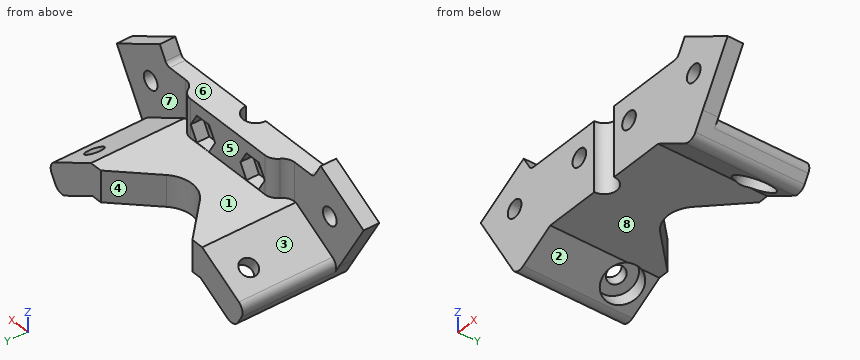
from build123d import *

# Parameters (mm, degrees)
SKETCH1_R                = 2.75
BOSS_EXTRUDE1_DEPTH      = 5
BOSS_EXTRUDE2_DEPTH      = 30
BOSS_EXTRUDE2_DEPTH_BACK = 5
BOSS_EXTRUDE3_DEPTH      = 12.320508
SKETCH5_R                = 4
CUT_EXTRUDE1_DEPTH       = 28.320508076
SKETCH7_R                = 2.75
CUT_EXTRUDE3_DEPTH       = 51.510942144
CUT_EXTRUDE4_START       = -4
SKETCH8_R                = 6
CUT_EXTRUDE4_DEPTH       = 47.510942144
SKETCH9_R                = 2.75
CUT_EXTRUDE5_DEPTH       = 10
CUT_EXTRUDE6_DEPTH       = 4
FILLET2_R                = 3


with BuildPart() as part:
    # Sketch1 → Boss-Extrude1 (new body)
    with BuildSketch(Plane(origin=(0, 0, 0), x_dir=(1, 0, 0), z_dir=(0, 1, 0))):
        with BuildLine():
            Line((-39.711904038, 0), (39.711904038, 0))
            Line((39.711904038, 0), (49.711904038, -17.320508076))
            Line((49.711904038, -17.320508076), (32.391395962, -27.320508076))
            Line((32.391395962, -27.320508076), (30.081994885, -23.320508076))
            ThreePointArc((30.081994885, -23.320508076), (29.349944078, -22.588457268), (28.349944078, -22.320508076))
            Line((28.349944078, -22.320508076), (-28.349944078, -22.320508076))
            ThreePointArc((-28.349944078, -22.320508076), (-29.349944078, -22.588457268), (-30.081994885, -23.320508076))
            Line((-30.081994885, -23.320508076), (-32.391395962, -27.320508076))
            Line((-32.391395962, -27.320508076), (-49.711904038, -17.320508076))
            Line((-49.711904038, -17.320508076), (-39.711904038, 0))
        make_face()
        with Locations(Location((-36.05165, -13.660254038, 0), (0, 0, 270))):  # turned: the seam where the file's is
            Circle(SKETCH1_R, mode=Mode.SUBTRACT)
        with Locations(Location((36.05165, -13.660254038, 0), (0, 0, 270))):  # turned: the seam where the file's is
            Circle(SKETCH1_R, mode=Mode.SUBTRACT)
    extrude(amount=BOSS_EXTRUDE1_DEPTH)

    # Sketch2 → Boss-Extrude2 (add, two sides)
    with BuildSketch(Plane(origin=(0, 5, 0), x_dir=(1, 0, 0), z_dir=(0, 1, 0))) as boss_extrude2_sk:
        with BuildLine():
            Line((-39.711904038, 0), (-22.391395962, -10))
            Line((-22.391395962, -10), (22.391395962, -10))
            Line((22.391395962, -10), (39.711904038, 0))
            Line((39.711904038, 0), (36.711904038, 5.196152423))
            ThreePointArc((36.711904038, 5.196152423), (34.890284962, 6.593929902), (32.613827826, 6.294228634))
            Line((32.613827826, 6.294228634), (21.711904038, 0))
            Line((21.711904038, 0), (-21.711904038, 0))
            Line((-21.711904038, 0), (-32.613827826, 6.294228634))
            ThreePointArc((-32.613827826, 6.294228634), (-34.890284962, 6.593929902), (-36.711904038, 5.196152423))
            Line((-36.711904038, 5.196152423), (-39.711904038, 0))
        make_face()
    extrude(amount=BOSS_EXTRUDE2_DEPTH)
    extrude(boss_extrude2_sk.sketch, amount=-BOSS_EXTRUDE2_DEPTH_BACK)

    # Sketch4 → Boss-Extrude3 (add)
    with BuildSketch(Plane.XY.offset(10)):
        with BuildLine():
            Line((-15, 9), (15, 9))
            ThreePointArc((15, 9), (17, 8.464101615), (18.464101615, 7))
            ThreePointArc((18.464101615, 7), (19.92820323, 5.535898385), (21.92820323, 5))
            Line((21.92820323, 5), (-21.92820323, 5))
            ThreePointArc((-21.92820323, 5), (-19.92820323, 5.535898385), (-18.464101615, 7))
            ThreePointArc((-18.464101615, 7), (-17, 8.464101615), (-15, 9))
        make_face()
    extrude(amount=BOSS_EXTRUDE3_DEPTH)

    # Sketch5 → Cut-Extrude1 (cut, through all)
    with BuildSketch(Plane(origin=(0, 0, 0), x_dir=(-1, 0, 0), z_dir=(0, 0, -1))):
        Circle(SKETCH5_R)
        with BuildLine():
            Line((-6.717514421, 23.282485579), (-18.435028843, 35))
            Line((-18.435028843, 35), (18.435028843, 35))
            Line((18.435028843, 35), (6.717514421, 23.282485579))
            ThreePointArc((6.717514421, 23.282485579), (0, 20.5), (-6.717514421, 23.282485579))
        make_face()
    extrude(amount=-CUT_EXTRUDE1_DEPTH, mode=Mode.SUBTRACT)

    # Sketch7 → Cut-Extrude3 (cut, through all)
    with BuildSketch(Plane(origin=(9.927976009, 0, 17.195758865), x_dir=(0.866025404, 0, -0.5), z_dir=(0.5, 0, 0.866025404))):
        with Locations((24.391517729, 27)):
            Circle(SKETCH7_R)
    cut_extrude3 = extrude(amount=-CUT_EXTRUDE3_DEPTH, mode=Mode.SUBTRACT)

    # Sketch8 → Cut-Extrude4 (cut, through all)
    with BuildSketch(Plane(origin=(9.927976009, 0, 17.195758865), x_dir=(0.866025404, 0, -0.5), z_dir=(0.5, 0, 0.866025404)).offset(CUT_EXTRUDE4_START)):
        with Locations((24.391517729, 27)):
            Circle(SKETCH8_R)
    cut_extrude4 = extrude(amount=-CUT_EXTRUDE4_DEPTH, mode=Mode.SUBTRACT)

    # Mirror1: Cut-Extrude3, Cut-Extrude4 across plane
    add(cut_extrude3.mirror(Plane(origin=(0, 0, 0), x_dir=(0, 0, 1), z_dir=(1, 0, 0))), mode=Mode.SUBTRACT)
    add(cut_extrude4.mirror(Plane(origin=(0, 0, 0), x_dir=(0, 0, 1), z_dir=(1, 0, 0))), mode=Mode.SUBTRACT)

    # Sketch9 → Cut-Extrude5 (cut, through all)
    with BuildSketch(Plane(origin=(0, 9, 0), x_dir=(1, 0, 0), z_dir=(0, 1, 0))):
        with Locations(Location((-10, -14.32050808, 0), (0, 0, 180))):  # turned: the seam where the file's is
            Circle(SKETCH9_R)
        with Locations(Location((10, -14.32050808, 0), (0, 0, 180))):  # turned: the seam where the file's is
            Circle(SKETCH9_R)
    extrude(amount=-CUT_EXTRUDE5_DEPTH, mode=Mode.SUBTRACT)

    # Sketch10 → Cut-Extrude6 (cut)
    with BuildSketch(Plane(origin=(0, 9, 0), x_dir=(1, 0, 0), z_dir=(0, 1, 0))):
        Polygon((-5.092522712, -14.32050808), (-7.546261356, -10.07050808), (-12.453738644, -10.07050808), (-14.907477288, -14.32050808), (-12.453738644, -18.57050808), (-7.546261356, -18.57050808), align=None)
        Polygon((5.092522712, -14.32050808), (7.546261356, -18.57050808), (12.453738644, -18.57050808), (14.907477288, -14.32050808), (12.453738644, -10.07050808), (7.546261356, -10.07050808), align=None)
    extrude(amount=-CUT_EXTRUDE6_DEPTH, mode=Mode.SUBTRACT)

    # Fillet2
    fillet2_edges = [part.edges().sort_by_distance(p)[0] for p in [
        (39.711904038, 20, 0),
        (-39.711904038, 20, 0),
    ]]
    fillet(fillet2_edges, radius=FILLET2_R)


solid = part.part
Design review of the part built by this model. Coordinates are the model's own, in mm. Face numbers are marked on the shaded views. A direction names the side the tool comes from. Coordinates: 2 decimals unless noted, no trailing zeros. Loops run counter-clockwise (first coordinate to the right, second up) from the corner with the lowest first, then second, coordinate; pieces in that order, holes last. Notation, with made-up numbers: (32, 73.25) - (69, 73.25) arc R21 cw to (69, 86.25) - close; hole circle Ø11 at (22.25, -10). An arc over 180 degrees is marked (long way). Use CSV: the item, a comma, the result in double quotes. Start each with the question number.
1. Add section D-D on x = 0. Give the boundary of the cut face in (y, z).
2. Add section C-C on y = 28. Count the separate pieces of the cut face and the enclosed holes in it, plus the area to 3 significant figures.
3. Mouldability with a two-part tool opening along X and no side actions: class the marked faces 1, 2, 3 and 4 as released by +X, released by -X, zero draft, split by the parting line, or undercut.
4. Clearance check with flat-ended pins moving along their axes: pin 1 (3 mm diameter, centred on x = 9, y = 7, fed in from +Z); pin 2 (6 mm diameter, centred on x = 12.5, y = 4, fed in from -Z); pin 3 (4 mm diameter, centred on x = -18.5, z = 22, fed in from +Y). State where each tip first meets the part, or that it passes through.
5. Add section A-A on y = 22. Give the boundary of the cut face in (x, z).
6. To check wall thickness, follow probe 1 along Z at (x, y) = (-10, 3); probe 2 along X at (y, z) = (28.5, 3); probe 3 along Y at (x, z) = (35, 4). State the ranges of each line that lie inside material, in increasing order.
7. For the marked faces 5, 6, 7 and 8, list the 3-axis set-ups (+Z, -Z, +X, -X, +Y, -Y) from which the entire face can be reached by the end or side of a thin tool; tool diameter is ignored.
8. Add section B-B on x = 10. Give the boundary of the cut face in (y, z).
Resolved:
1,outline,"(4, 0) - (20.5, 0) - (20.5, 10) - (9, 10) - (9, 22.32) - (4, 22.32) - close"
2,separate pieces,"4"
2,enclosed holes,"0"
2,area,"366 mm2"
3,face 1,"zero draft"
3,face 2,"undercut"
3,face 3,"released by -X"
3,face 4,"undercut"
4,pin 1,"z = 22.32"
4,pin 2,"z = 0"
4,pin 3,"y = 8.71"
5,outline,"(-38.21, -2.6) - (-36.71, -5.2) arc R3 ccw to (-32.61, -6.29) - (-29.42, -4.45) - (-31.92, -0.12) - (-26.18, 3.19) - (-23.68, -1.14) - (-21.71, 0) - (-5.12, 0) - (-5.12, 10) - (-22.39, 10) - (-37.11, 1.5) arc R3 ccw to start; (5.12, 0) - (21.71, 0) - (23.68, -1.14) - (26.18, 3.19) - (31.92, -0.12) - (29.42, -4.45) - (32.61, -6.29) arc R3 ccw to (36.71, -5.2) - (38.21, -2.6) arc R3 ccw to (37.11, 1.5) - (22.39, 10) - (5.12, 10) - close"
6,probe 1,"0 to 11.57, 17.07 to 22.32"
6,probe 2,"-34.52 to -32.56, -27.24 to -26.52, -23.19 to -11.94, 11.94 to 23.19, 26.52 to 27.24, 32.56 to 34.52"
6,probe 3,"0 to 5"
7,face 5,"+Z, +X, -X, +Y"
7,face 6,"+Z, +Y, -Y"
7,face 7,"+Z, +X, +Y"
7,face 8,"-Z, +Y, -Y"
8,outline,"(0, 0) - (26.56, 0) - (26.56, 10) - (9, 10) - (9, 10.07) - (5, 10.07) - (5, 11.57) - (0, 11.57) - close; (0, 17.07) - (5, 17.07) - (5, 18.57) - (9, 18.57) - (9, 22.32) - (0, 22.32) - close"
